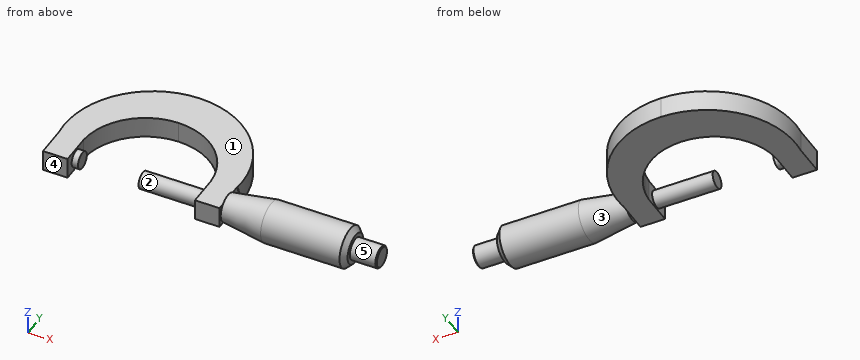
from build123d import *

# Parameters (mm, degrees)
BOSS_EXTRUDE1_DEPTH = 2.54
SKETCH3_R           = 4.865340766
BOSS_EXTRUDE2_DEPTH = 30.48
CHAMFER5_SIZE       = 1.27
SKETCH5_R           = 2.590082511
BOSS_EXTRUDE3_DEPTH = 6.35
CHAMFER6_SIZE       = 0.254
SKETCH6_R           = 2.032
BOSS_EXTRUDE4_DEPTH = 1.524
SKETCH7_R           = 2.032
BOSS_EXTRUDE5_DEPTH = 14.478


with BuildPart() as part:
    # Sketch2 → Boss-Extrude1 (new body, symmetric)
    with BuildSketch(Plane.XY):
        with BuildLine():
            Line((-21.110510204, -3.916551019), (-15.24, -3.916551019))
            Line((-15.24, -3.916551019), (-15.24, 3.470183675))
            ThreePointArc((-15.24, 3.470183675), (-10.479530006, 13.693144777), (0, 17.858533009))
            Line((0, 17.858533009), (0, 27.35528296))
            ThreePointArc((0, 27.35528296), (-15.938566505, 20.170697643), (-21.110510204, 3.470183675))
            Line((-21.110510204, 3.470183675), (-21.110510204, -3.916551019))
        make_face()
    boss_extrude1 = extrude(amount=BOSS_EXTRUDE1_DEPTH, both=True)

    # Mirror1: Boss-Extrude1 across plane
    add(boss_extrude1.mirror(Plane(origin=(0, 0, 0), x_dir=(0, 0, 1), z_dir=(1, 0, 0))))

    # Sketch3 → Boss-Extrude2 (add)
    with BuildSketch(Plane(origin=(21.110510204, 0, 0), x_dir=(0, 0, -1), z_dir=(1, 0, 0))):
        Circle(SKETCH3_R)
    extrude(amount=BOSS_EXTRUDE2_DEPTH)

    # Sketch4 → Cut-Revolve1 (revolve, cut)
    with BuildSketch(Plane.XY):
        Polygon((21.110510204, 3.342420759), (21.110510204, 4.865340766), (31.445897446, 4.865340766), align=None)
    revolve(axis=Axis((51.590510204, 0, 0), (-1, 0, 0)), mode=Mode.SUBTRACT)

    # Chamfer5
    chamfer5_edges = [part.edges().sort_by_distance(p)[0] for p in [
        (51.590510204, 0, 4.865340766),
    ]]
    chamfer(chamfer5_edges, length=CHAMFER5_SIZE)

    # Sketch5 → Boss-Extrude3 (add)
    with BuildSketch(Plane(origin=(51.590510204, 0, 0), x_dir=(0, 0, -1), z_dir=(1, 0, 0))):
        Circle(SKETCH5_R)
    extrude(amount=BOSS_EXTRUDE3_DEPTH)

    # Chamfer6
    chamfer6_edges = [part.edges().sort_by_distance(p)[0] for p in [
        (57.940510204, 0, 2.590082511),
    ]]
    chamfer(chamfer6_edges, length=CHAMFER6_SIZE)

    # Sketch6 → Boss-Extrude4 (add)
    with BuildSketch(Plane(origin=(-15.24, 0, 0), x_dir=(0, 0, -1), z_dir=(1, 0, 0))):
        Circle(SKETCH6_R)
    extrude(amount=BOSS_EXTRUDE4_DEPTH)

    # Sketch7 → Boss-Extrude5 (add)
    with BuildSketch(Plane.ZY.offset(-15.24)):
        Circle(SKETCH7_R)
    extrude(amount=BOSS_EXTRUDE5_DEPTH)


solid = part.part
Source: CAD feature listing. Evaluate the final solid. Frame: model axes, mm. Face numbers are marked on the shaded views. A direction names the side the tool comes from. Give positions to 0.01 mm unless a question says otherwise; leave off trailing zeros. Write each loop counter-clockwise with the first axis right and the second up, starting at its lowest first coordinate (ties: lowest second). Pieces come first, ordered by that corner, then holes. Notation, with made-up numbers: M 81,83.5 L 121,83.5 A16 cw 121,112.5 Z; hole C -24.75,-31 d8. An arc over 180 degrees is marked long. Return JSON: item names as keys, results as strings. Group by question number.
1) Cut plane D-D, the plane y = 17. Output: boundary loops of the cut face in (x, z), plus the area to 3 significant figures.
2) Set-up query: the marked faces 3, 4 and 5. Return all of +Z, -Z, +X, -X, +Y, -Y with unobstructed straight access to the full face (end or side cutting, diameter ignored); none if empty.
3) Material intervals for line 1 along X through (y, z) = (6.5, 2.25); line 2 along Z through (x, y) = (-15.5, 7); line 3 along X through (y, z) = (7, -2), sorted ascending. Write a range as [from, to].
4) Pin query (flat end, axial travel): P1, Ø2, axis at y = 0.5, z = 1, coming from the -X side; P2, Ø1, axis at y = 4.5, z = 1, coming from the -X side; P3, Ø4, axis at y = 4.5, z = -0.5, coming from the +X side; P4, Ø2, axis at x = 24, y = 7, coming from the +Z side. Return the tip coordinate at first contact, or that it passes through.
5) Pull-direction query (X, two-part tool) for the marked faces 1 and 2; classes: pulls with the +X half, pulls with the -X half, needs draft (parallel to the pull), parting line crosses it, or undercut.
6) Cut plane B-B, the plane x = 14. Output: boundary loops of the cut face in (y, z), plus the area to 3 significant figures.
Recorded:
{
 "1": {"outline": "M -18.26,-2.54 L -5.05,-2.54 L -5.05,2.54 L -18.26,2.54 Z; M 5.05,-2.54 L 18.26,-2.54 L 18.26,2.54 L 5.05,2.54 Z", "area": "134 mm²"},
 "2": {"face 3": "none", "face 4": "+Z, -Z, -X, -Y", "face 5": "+X"},
 "3": {"line 1": "x = [-21.27, -14.76], [14.76, 21.27]", "line 2": "z = [-2.54, 2.54]", "line 3": "x = [-21.25, -14.62], [14.62, 21.25]"},
 "4": {"P1": "stops at x = -21.11", "P2": "stops at x = -21.24", "P3": "stops at x = 57.75", "P4": "passes through"},
 "5": {"face 1": "needs draft", "face 2": "undercut"},
 "6": {"outline": "C 0,0 d4.06; M 8.68,-2.54 L 22.1,-2.54 L 22.1,2.54 L 8.68,2.54 Z", "area": "81.1 mm²"}
}
